from build123d import *

# Parameters (mm, degrees)
SKETCH_R     = 2
PAD_DEPTH    = 2
SKETCH001_R  = 2
PAD001_DEPTH = 2
FILLET_R     = 1.9


with BuildPart() as part:
    # Sketch → Pad (new body)
    with BuildSketch(Plane.XY):
        Polygon((13, 3), (13, -3), (10.21455, -5), (6.78545, -5), (4, -3), (0, -3), (0, 3), (4, 3), (6.78545, 5), (10.21455, 5), align=None)
        with Locations((8.5, 0)):
            Circle(SKETCH_R, mode=Mode.SUBTRACT)
    extrude(amount=PAD_DEPTH)

    # Sketch001 → Pad001 (new body)
    with BuildSketch(Plane(origin=(0, 0, 0), x_dir=(0, -1, 0), z_dir=(-1, 0, 0))):
        Polygon((-3, 0), (3, 0), (3, -2), (5.636039, -4.636039), (5.636039, -8.363961), (3, -11), (-3, -11), (-5.636039, -8.363961), (-5.636039, -4.636039), (-3, -2), align=None)
        with Locations((0, -6.5)):
            Circle(SKETCH001_R, mode=Mode.SUBTRACT)
    extrude(amount=-PAD001_DEPTH)

    # Fillet
    fillet_edges = [part.edges().sort_by_distance(p)[0] for p in [
        (2, 0, 0),
        (0, 0, 2),
    ]]
    fillet(fillet_edges, radius=FILLET_R)


solid = part.part
Design review of the part built by this model. Coordinates are the model's own, in mm. A direction names the side the tool comes from. Round coordinates to 2 decimals unless told otherwise and drop trailing zeros. Loops run counter-clockwise (first coordinate to the right, second up) from the corner with the lowest first, then second, coordinate; pieces in that order, holes last. Notation, with made-up numbers: (21, -20.5) - (45, -20.5) arc R20 cw to (45, -6.5) - close; hole circle Ø2 at (4.25, 18.25). An arc over 180 degrees is marked (long way). One line per item, written item: value. Start each with the question number.
1) Consider section B-B on x = 8.5. Give the boundary of the cut face in (y, z), then the cut area to 3 significant figures.
2) For faces 1 (the flat face through (2, 3, 0)), 2 (the flat face through (2, -3, 0)), 3 (the cylindrical face through (0.542, 0.042, 1.429)), 4 (the flat face through (2, 0, -4)), list the 3-axis set-ups (+Z, -Z, +X, -X, +Y, -Y) from which the entire face can be reached by the end or side of a thin tool; tool diameter is ignored.
3) Consider section D-D on z = -4. Give the boundary of the cut face in (x, y).
4) To check wall thickness, follow L1, parallel to Z at x = 5, y = 1.75; L2, parallel to Y at x = 8.75, z = 1. State the ranges of each line that lie inside material, in increasing order. Write a range as from..to.
5) Consider section C-C on z = -6.5. Give the boundary of the cut face in (x, y), then the cut area to 3 significant figures.
6) Insertion check: pin 1 Ø2 at (x, z) = (2.5, 0.5) entering from -Y; pin 2 Ø1.5 at (x, z) = (10.5, 0) entering from +Y; pin 3 Ø6 at (x, z) = (1.5, -2.5) entering from +Y; pin 4 Ø5 at (x, z) = (5, -0.5) entering from -Y. Each pin has a flat end and moves straight along its axis. Give the tip position at first contact, or say it passes through.
7) Consider section A-A on y = 0. Give the boundary of the cut face in (x, z), then the cut area to 3 significant figures.
Reported:
1. outline: (-5, 0) - (-2, 0) - (-2, 2) - (-5, 2) - close; (2, 0) - (5, 0) - (5, 2) - (2, 2) - close
1. area: 12.0 mm^2
2. face 1: +Z, -X, +Y
2. face 2: +Z, -X, -Y
2. face 3: +Z, -X, +Y, -Y
2. face 4: -Z, +X, +Y, -Y
3. outline: (0, -5) - (2, -5) - (2, 5) - (0, 5) - close
4. L1: z = 0..2
4. L2: y = -5..-1.98, 1.98..5
5. outline: (0, -5.64) - (2, -5.64) - (2, -2) - (0, -2) - close; (0, 2) - (2, 2) - (2, 5.64) - (0, 5.64) - close
5. area: 14.5 mm^2
6. pin 1: stops at y = -3
6. pin 2: stops at y = 5
6. pin 3: stops at y = 5.64
6. pin 4: stops at y = -5
7. outline: (0, -11) - (2, -11) - (2, -8.5) - (0, -8.5) - close; (0, -4.5) - (2, -4.5) - (2, -1.9) arc R1.9 cw to (3.9, 0) - (6.5, 0) - (6.5, 2) - (1.9, 2) arc R1.9 ccw to (0, 0.1) - close; (10.5, 0) - (13, 0) - (13, 2) - (10.5, 2) - close
7. area: 32.0 mm^2
